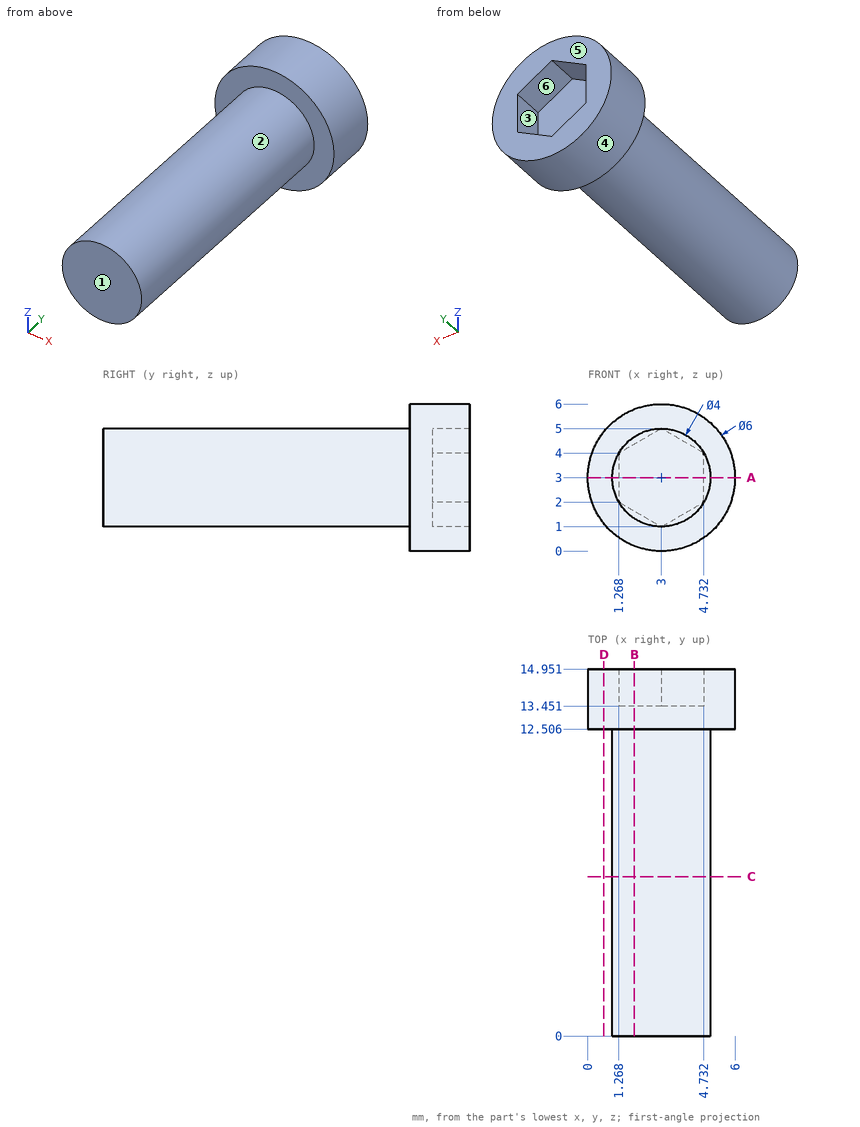
Print and shaded views of the part. All mm, measured from the part's lowest x, y and z. A direction names the side the tool comes from. Coordinates: 2 decimals unless noted, no trailing zeros. Loops run counter-clockwise (first coordinate to the right, second up) from the corner with the lowest first, then second, coordinate; pieces in that order, holes last. Notation, with made-up numbers: (-39.5, 18.5) - (-31.5, 18.5) arc R16 cw to (-31.5, 24.5) - close; hole circle Ø4 at (24, 63). An arc over 180 degrees is marked (long way). Write item = value, one per line. Start each with the question number.
Item 1: Cut at B-B, the plane x = 1.9. Give the cut face in (y, z) (1 decimal).
Item 2: Cut at D-D, the plane x = 0.65. Give the cut face in (y, z) (3 decimals).
Item 3: Mould opens along Z. For the marked faces 4, 5 and 6 say: released by +Z, released by -Z, zero draft, split by the parting line, or undercut.
Item 4: Cut at C-C, the plane y = 6.5. Give the cut face in (x, z), and give its area (3 significant figures).
Item 5: Flat gauge pins, fed straight in: pin 1 Ø3 at (x, z) = (3, 3.5) entering from +Y; pin 2 Ø1.5 at (x, y) = (4, 11) entering from -Z; pin 3 Ø1 at (y, z) = (3.5, 4.5) entering from +X; pin 4 Ø1 at (x, z) = (2.5, 3) entering from +Y. Where does each tip first touch, or does it go through?
Item 6: Wall check: L1, parallel to X at y = 5.75, z = 2.95; L2, parallel to Y at x = 2.35, z = 1.8; L3, parallel to X at y = 1.25, z = 4. Give the ranges that are in metal, low to high. Write a range as from..to.
Item 7: Cut at A-A, the plane z = 3. Give the cut face in (x, y), and give its area (3 significant figures).
Item 8: 3-axis set-ups, long thin cutter, end or side, ignore diameter. For the marked faces 1, 2 and 3: which of +Z, -Z, +X, -X, +Y, -Y reach the whole face in a straight line?
The answers:
q1.outline = (0, 1.3) - (12.5, 1.3) - (12.5, 0.2) - (15, 0.2) - (15, 1.6) - (13.5, 1.6) - (13.5, 4.4) - (15, 4.4) - (15, 5.8) - (12.5, 5.8) - (12.5, 4.7) - (0, 4.7) - close
q2.outline = (12.506, 1.135) - (14.951, 1.135) - (14.951, 4.865) - (12.506, 4.865) - close
q3.face_4 = split by the parting line
q3.face_5 = zero draft
q3.face_6 = undercut
q4.outline = circle Ø4 at (3, 3)
q4.area = 12.6 mm2
q5.pin_1 = 14.95
q5.pin_2 = 1.02
q5.pin_3 = 4.73
q5.pin_4 = 13.45
q6.L1 = 1..5
q6.L2 = 0..13.45
q6.L3 = 1.27..4.73
q7.outline = (0, 12.51) - (1, 12.51) - (1, 0) - (5, 0) - (5, 12.51) - (6, 12.51) - (6, 14.95) - (4.73, 14.95) - (4.73, 13.45) - (1.27, 13.45) - (1.27, 14.95) - (0, 14.95) - close
q7.area = 59.5 mm2
q8.face_1 = +Z, -Z, +X, -X, -Y
q8.face_2 = -Y
q8.face_3 = +Y
